Can you work these out from the model? Positions are in its coordinate system, mm. A direction names the side the tool comes from. Give positions to 0.01 mm unless a question says otherwise; leave off trailing zeros. Loops run counter-clockwise (first coordinate to the right, second up) from the corner with the lowest first, then second, coordinate; pieces in that order, holes last. Notation, with made-up numbers: M 57.25,-7 L 89.25,-7 A27 ccw 89.25,31 Z; hole C 73,20.25 d5. An arc over 180 degrees is marked long. Answer as a JSON object with one key per item and string values.
```python
from build123d import *

# Parameters (mm, degrees)
F0_W     = 32
F0_H     = 16
F1_DEPTH = 9
F2_R     = 2.5
F3_DEPTH = 1.5
F4_W     = 29
F4_H     = 13
F5_DEPTH = 7.5
F6_R     = 3
F7_DEPTH = 7.5
F8_R     = 2.25
F9_DEPTH = 7.5


with BuildPart() as f1:
    # F0 (on Top) → F1 (new body)
    with BuildSketch(Plane.XY):
        with Locations((16, 8)):
            Rectangle(F0_W, F0_H)
    extrude(amount=F1_DEPTH)

    # F2 (on face) → F3 (join)
    with BuildSketch(Plane.XY.offset(9)):
        with Locations((4, 4.107877)):
            Circle(F2_R)
        with Locations((4, 12.107877)):
            Circle(F2_R)
        with Locations((12, 12.107877)):
            Circle(F2_R)
        with Locations((12, 4.107877)):
            Circle(F2_R)
        with Locations((20, 12.107877)):
            Circle(F2_R)
        with Locations((20, 4.107877)):
            Circle(F2_R)
        with Locations((28, 4.107877)):
            Circle(F2_R)
        with Locations((28, 12.107877)):
            Circle(F2_R)
    extrude(amount=F3_DEPTH)

    # F4 (on face) → F5 (cut)
    with BuildSketch(Plane(origin=(0, 0, 0), x_dir=(1, 0, 0), z_dir=(0, 0, -1))):
        with Locations((16, -8)):
            Rectangle(F4_W, F4_H)
    extrude(amount=-F5_DEPTH, mode=Mode.SUBTRACT)

    # F6 (on face) → F7 (join)
    with BuildSketch(Plane(origin=(0, 0, 7.5), x_dir=(1, 0, 0), z_dir=(0, 0, -1))):
        with Locations((8, -8)):
            Circle(F6_R)
        with Locations((16, -8)):
            Circle(F6_R)
        with Locations((24, -8)):
            Circle(F6_R)
    extrude(amount=F7_DEPTH)

    # F8 (on face) → F9 (cut)
    with BuildSketch(Plane(origin=(0, 0, 0), x_dir=(1, 0, 0), z_dir=(0, 0, -1))):
        with Locations((8, -8)):
            Circle(F8_R)
        with Locations((16, -8)):
            Circle(F8_R)
        with Locations((24, -8)):
            Circle(F8_R)
    extrude(amount=-F9_DEPTH, mode=Mode.SUBTRACT)


solid = f1.part
```
1) Please list where these lines run through material, in increasing order: line 1 along Y through (x, z) = (8, 6); line 2 along X through (y, z) = (4, 0.5); line 3 along Y through (x, z) = (17, 5.5). Write a range as from..to.
Answer list:
{"line 1": "0..1.5, 5..5.75, 10.25..11, 14.5..16", "line 2": "0..1.5, 30.5..32", "line 3": "0..1.5, 5.17..5.98, 10.02..10.83, 14.5..16"}
2) If we mould it in two halves opening along X, with no side actions, what happens to faces 4 (the flat face through (32, 8, 4)), 5 (the cylindrical face through (6.34, 6.48, 3.7)), 6 (the cylindrical face through (26.016, 2.587, 9.74)), 7 (the flat face through (0, 8, 4))? For each: +X half, -X half, draft (parallel to the pull), parting line (faces both ways), or undercut.
Answer list:
{"face 4": "+X half", "face 5": "undercut", "face 6": "undercut", "face 7": "-X half"}
3) For faces 1 (the flat face through (30.5, 8, 4)), 2 (the flat face through (16, 8, 9)), 3 (the flat face through (28, 4, 10.5)), which set-ups out of +Z, -Z, +X, -X, +Y, -Y let a thin tool reach every point of the face, with its end or its side?
Answer list:
{"face 1": "-Z", "face 2": "+Z", "face 3": "+Z, +X, -X, +Y, -Y"}
4) Will these pins go through, and if not, where does the flat tip stop? pin 1 Ø2.5 at (x, y) = (16, 8) entering from -Z; pin 2 Ø7 at (x, y) = (24, 8) entering from +Z.
Answer list:
{"pin 1": "z = 7.5", "pin 2": "z = 10.5"}
5) Suppose I cut it at A-A, the plane z = 4.5. Write out the boundary of the cut face in (x, y), and give its area (3 significant figures).
Answer list:
{"outline": "M 0,0 L 32,0 L 32,16 L 0,16 Z; C 8,8 d6; C 16,8 d6; C 24,8 d6; hole M 1.5,1.5 L 30.5,1.5 L 30.5,14.5 L 1.5,14.5 Z; hole C 8,8 d4.5; hole C 16,8 d4.5; hole C 24,8 d4.5", "area": "172 mm^2"}
6) Suppose I cut it at B-B, the plane x = 28. Write out the boundary of the cut face in (y, z), and give its area (3 significant figures).
Answer list:
{"outline": "M 0,0 L 1.5,0 L 1.5,7.5 L 14.5,7.5 L 14.5,0 L 16,0 L 16,9 L 14.61,9 L 14.61,10.5 L 9.61,10.5 L 9.61,9 L 6.61,9 L 6.61,10.5 L 1.61,10.5 L 1.61,9 L 0,9 Z", "area": "61.5 mm^2"}
7) Suppose I cut it at D-D, the plane x = 16. Write out the boundary of the cut face in (y, z).
Answer list:
{"outline": "M 0,0 L 1.5,0 L 1.5,7.5 L 5,7.5 L 5,0 L 5.75,0 L 5.75,7.5 L 10.25,7.5 L 10.25,0 L 11,0 L 11,7.5 L 14.5,7.5 L 14.5,0 L 16,0 L 16,9 L 0,9 Z"}
